from build123d import *

# Parameters (mm, degrees)
F1_DEPTH = 65.278
F2_W     = 22.147088
F2_H     = 17.75202
F3_DEPTH = 25.4


with BuildPart() as f1:
    # F0 (on Front) → F1 (new body)
    with BuildSketch(Plane.XZ):
        Polygon((-18.030003, 24.418592), (-39.609224, 24.418592), (-39.609224, -24.418592), (39.609224, -24.418592), (39.609224, 24.418592), (17.462136, 24.418592), (17.462136, 0), (-11.215512, 0), (-18.030003, 0), align=None)
    extrude(amount=F1_DEPTH)

    # F2 (on face) → F3 (cut)
    with BuildSketch(Plane.XY.offset(24.418592)):
        with Locations((28.53568, -33.411176)):
            Rectangle(F2_W, F2_H)
    extrude(amount=-F3_DEPTH, mode=Mode.SUBTRACT)


solid = f1.part
For this review, take the finished solid that the model builds, in its own axes (mm). A direction names the side the tool comes from. Give positions to 0.01 mm unless a question says otherwise; leave off trailing zeros. Loops run counter-clockwise (first coordinate to the right, second up) from the corner with the lowest first, then second, coordinate; pieces in that order, holes last.
Item 1: Take a section at C-C, the plane y = -32. State the section outline as (x, z) points, and give its area (3 significant figures).
Item 2: Take a section at B-B, the plane x = 28. State the section outline as (y, z) points, and give its area (3 significant figures).
Item 3: For line 1 along X through (y, z) = (-61.5, 20.5); line 2 along Z through (x, y) = (4.5, -56); line 3 along Y through (x, z) = (35, 2), list the stretches that pass through material, from the lowest coordinate up.
Item 4: Draft analysis for pull direction Y (two halves, no side actions). For faces 1 (the flat face through (28, -24.535, 12)), 2 (the flat face through (-1, -65.278, -5)), 3 (the flat face through (17.462, -54, 12)), state which applies: +Y half, -Y half, draft (parallel to the pull), parting line (faces both ways), or undercut.
Item 5: Take a section at A-A, the plane z = 14. State the section outline as (x, y) points, and give its area (3 significant figures).
Item 6: Insertion check: pin 1 (17.5 mm diameter, centred on x = -5.5, y = -40.5, fed in from +Z); pin 2 (9 mm diameter, centred on x = 28.5, y = -31.5, fed in from +Z); pin 3 (0.5 mm diameter, centred on y = -29.5, z = -0.5, fed in from +X). Each pin has a flat end and moves straight along its axis. Give the tip position at first contact, or say it passes through.
Item 7: Tool access review of faces 4 (the flat face through (28, -33, -0.981)), 5 (the flat face through (29, -54, 24.419)), 6 (the flat face through (17.462, -12, 12)): name each direction out of +Z, -Z, +X, -X, +Y, -Y from which nothing blocks a thin tool from reaching the whole face with its end or side.
Item 8: Take a section at D-D, the plane x = -1. State the section outline as (y, z) points.
Calculated:
1. outline: (-39.61, -24.42) - (39.61, -24.42) - (39.61, -0.98) - (17.46, -0.98) - (17.46, 0) - (-18.03, 0) - (-18.03, 24.42) - (-39.61, 24.42) - close
1. area: 2,440 mm2
2. outline: (-65.28, -24.42) - (0, -24.42) - (0, 24.42) - (-24.54, 24.42) - (-24.54, -0.98) - (-42.29, -0.98) - (-42.29, 24.42) - (-65.28, 24.42) - close
2. area: 2,740 mm2
3. line 1: x = -39.61 to -18.03, 17.46 to 39.61
3. line 2: z = -24.42 to 0
3. line 3: y = -65.28 to -42.29, -24.54 to 0
4. face 1: undercut
4. face 2: -Y half
4. face 3: draft
5. outline: (-39.61, -65.28) - (-18.03, -65.28) - (-18.03, 0) - (-39.61, 0) - close; (17.46, -65.28) - (39.61, -65.28) - (39.61, -42.29) - (17.46, -42.29) - close; (17.46, -24.54) - (39.61, -24.54) - (39.61, 0) - (17.46, 0) - close
5. area: 2,460 mm2
6. pin 1: stops at z = 0
6. pin 2: stops at z = -0.98
6. pin 3: stops at x = 17.46
7. face 4: +Z, +X
7. face 5: +Z, +X, -X, +Y, -Y
7. face 6: +Z, +Y, -Y
8. outline: (-65.28, -24.42) - (0, -24.42) - (0, 0) - (-65.28, 0) - close
